Could you check a few things on this model? Use its own coordinates, in mm. Coordinates: 2 decimals unless noted, no trailing zeros. Order: outer loops, then holes, each group sorted by start corner. A loop starts at its lowest first (then second) coordinate and runs counter-clockwise, first axis right, second up. Notation, with made-up numbers: M -22,33 L 2,33 A21 ccw 2,43 Z; hole C 29.5,56.5 d5. An arc over 180 degrees is marked long. One line per question, with ' | ' between items. Start each with the question number.
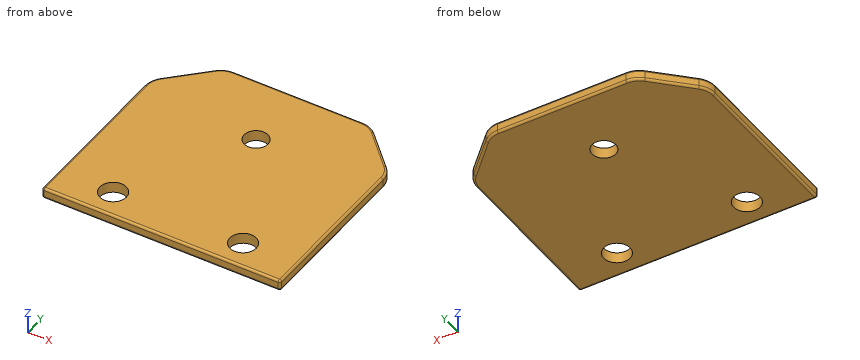
from build123d import *

# Parameters (mm, degrees)
SKETCH1_R           = 6.1
SKETCH1_R_2         = 5.5
BOSS_EXTRUDE1_DEPTH = 5
FILLET1_R           = 10
FILLET2_R           = 1


with BuildPart() as part:
    # Sketch1 → Boss-Extrude1 (new body)
    with BuildSketch(Plane.XY):
        Polygon((0, 0), (110, 0), (110, 80), (88.786796564, 101.213203436), (21.213203436, 101.213203436), (0, 80), align=None)
        with Locations((25, 12.5)):
            Circle(SKETCH1_R, mode=Mode.SUBTRACT)
        with Locations((85, 12.5)):
            Circle(SKETCH1_R, mode=Mode.SUBTRACT)
        with Locations((55, 70)):
            Circle(SKETCH1_R_2, mode=Mode.SUBTRACT)
    extrude(amount=BOSS_EXTRUDE1_DEPTH)

    # Fillet1
    fillet1_edges = [part.edges().sort_by_distance(p)[0] for p in [
        (110, 80, 2.5),
        (0, 80, 2.5),
        (21.213203436, 101.213203436, 2.5),
        (88.786796564, 101.213203436, 2.5),
    ]]
    fillet(fillet1_edges, radius=FILLET1_R)

    # Fillet2
    fillet2_edges = [part.edges().sort_by_distance(p)[0] for p in [
        (110, 37.928932188, 0),
        (55, 0, 0),
        (0, 37.928932188, 0),
        (110, 0, 2.5),
        (0, 0, 2.5),
        (0, 37.928932188, 5),
        (55, 0, 5),
        (99.393398282, 90.606601718, 0),
        (99.393398282, 90.606601718, 5),
        (10.606601718, 90.606601718, 0),
        (55, 101.213203436, 0),
        (21.528504736, 100.451998761, 0),
        (110, 37.928932188, 5),
        (0.761204675, 79.6846987, 0),
        (88.471495264, 100.451998761, 0),
        (109.238795325, 79.6846987, 0),
        (55, 101.213203436, 5),
        (10.606601718, 90.606601718, 5),
        (21.528504736, 100.451998761, 5),
        (0.761204675, 79.6846987, 5),
        (88.471495264, 100.451998761, 5),
        (109.238795325, 79.6846987, 5),
    ]]
    fillet(fillet2_edges, radius=FILLET2_R)


solid = part.part
(1) For P1, Ø11, axis at x = 85, y = 12.5, coming from the +Z side, with a flat end and sliding along its axis, tell me the tip position at first contact or that it passes through.
(2) If I drill on line 1 along Y through (x, z) = (25, 2); line 2 along Y through (x, z) = (55, 3.2); line 3 along X through (y, z) = (11.5, 1.6), over which ranges is the centre line in solid material (lowest first)? Write a range as from..to.
(3) Imagine slicing it at A-A, the plane z = 2.3. Write out the boundary of the cut face in (x, y).
(4) Imagine slicing it at B-B, the plane x = 55. Write out the boundary of the cut face in (y, z).
(5) Imagine slicing it at D-D, the plane y = 10.5. Write out the boundary of the cut face in (x, z), plus the area to 3 significant figures.
(6) Imagine slicing it at C-C, the plane y = 70. Write out the boundary of the cut face in (x, z), plus the area to 3 significant figures.
Answers:
1) P1: through
2) line 1: 0..6.4, 18.6..101.21 | line 2: 0..64.5, 75.5..101.21 | line 3: 0..18.98, 31.02..78.98, 91.02..110
3) outline: M 0,1 A1 ccw 1,0 L 109,0 A1 ccw 110,1 L 110,75.86 A10 ccw 107.07,82.93 L 91.72,98.28 A10 ccw 84.64,101.21 L 25.36,101.21 A10 ccw 18.28,98.28 L 2.93,82.93 A10 ccw 0,75.86 Z; hole C 25,12.5 d12.2; hole C 55,70 d11; hole C 85,12.5 d12.2
4) outline: M 0,1 A1 ccw 1,0 L 64.5,0 L 64.5,5 L 1,5 A1 ccw 0,4 Z; M 75.5,0 L 100.21,0 A1 ccw 101.21,1 L 101.21,4 A1 ccw 100.21,5 L 75.5,5 Z
5) outline: M 0,1 A1 ccw 1,0 L 19.24,0 L 19.24,5 L 1,5 A1 ccw 0,4 Z; M 30.76,0 L 79.24,0 L 79.24,5 L 30.76,5 Z; M 90.76,0 L 109,0 A1 ccw 110,1 L 110,4 A1 ccw 109,5 L 90.76,5 Z | area: 434 mm²
6) outline: M 0,1 A1 ccw 1,0 L 49.5,0 L 49.5,5 L 1,5 A1 ccw 0,4 Z; M 60.5,0 L 109,0 A1 ccw 110,1 L 110,4 A1 ccw 109,5 L 60.5,5 Z | area: 494 mm²
